Could you check a few things on this model? Use its own coordinates, in mm. Face numbers are marked on the shaded views. A direction names the side the tool comes from. Coordinates: 2 decimals unless noted, no trailing zeros. Loops run counter-clockwise (first coordinate to the right, second up) from the corner with the lowest first, then second, coordinate; pieces in that order, holes last. Notation, with made-up numbers: M 43.25,82.5 L 89.25,82.5 A13 ccw 89.25,86.5 Z; hole C 67,85 d6. An arc over 180 degrees is marked long. Return JSON: item names as keys, results as strings. Group by question number.
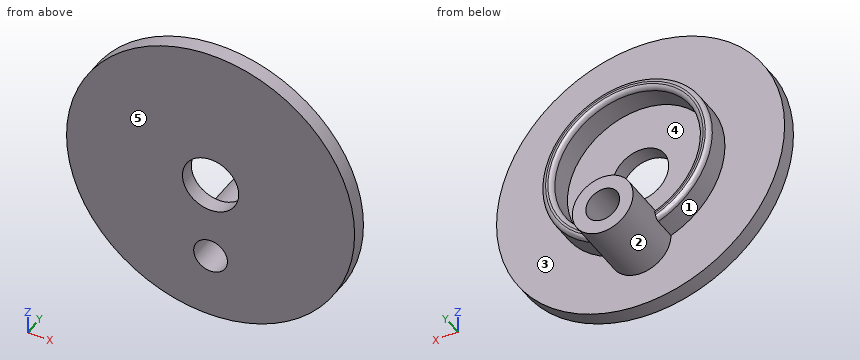
from build123d import *

# Parameters (mm, degrees)
SKETCH2_R           = 64
BOSS_EXTRUDE1_DEPTH = 7
SKETCH3_R           = 37.5
SKETCH3_R_2         = 32.5
BOSS_EXTRUDE2_DEPTH = 12
SKETCH4_R           = 12.5
CUT_EXTRUDE1_DEPTH  = 8
FILLET1_R           = 2
SKETCH5_R           = 13.5
BOSS_EXTRUDE3_DEPTH = 30
SKETCH7_R           = 7.5
CUT_EXTRUDE2_DEPTH  = 38


with BuildPart() as part:
    # Sketch2 → Boss-Extrude1 (new body)
    with BuildSketch(Plane(origin=(0, 0, 0), x_dir=(1, 0, 0), z_dir=(0, 1, 0))):
        Circle(SKETCH2_R)
    extrude(amount=BOSS_EXTRUDE1_DEPTH)

    # Sketch3 → Boss-Extrude2 (add)
    with BuildSketch(Plane(origin=(0, 7, 0), x_dir=(1, 0, 0), z_dir=(0, 1, 0))):
        Circle(SKETCH3_R)
        Circle(SKETCH3_R_2, mode=Mode.SUBTRACT)
    extrude(amount=BOSS_EXTRUDE2_DEPTH)

    # Sketch4 → Cut-Extrude1 (cut, through all)
    with BuildSketch(Plane(origin=(0, 7, 0), x_dir=(1, 0, 0), z_dir=(0, 1, 0))):
        Circle(SKETCH4_R)
    extrude(amount=-CUT_EXTRUDE1_DEPTH, mode=Mode.SUBTRACT)

    # Fillet1
    fillet1_edges = [part.edges().sort_by_distance(p)[0] for p in [
        (-37.5, 19, 0),
        (-32.5, 19, 0),
    ]]
    fillet(fillet1_edges, radius=FILLET1_R)

    # Sketch5 → Boss-Extrude3 (add)
    with BuildSketch(Plane(origin=(0, 7, 0), x_dir=(1, 0, 0), z_dir=(0, 1, 0))):
        with Locations((0, 35)):
            Circle(SKETCH5_R)
    extrude(amount=BOSS_EXTRUDE3_DEPTH)

    # Sketch7 → Cut-Extrude2 (cut, through all)
    with BuildSketch(Plane(origin=(0, 37, 0), x_dir=(1, 0, 0), z_dir=(0, 1, 0))):
        with Locations((0, 35)):
            Circle(SKETCH7_R)
    extrude(amount=-CUT_EXTRUDE2_DEPTH, mode=Mode.SUBTRACT)


solid = part.part
(1) Will these pins go through, and if not, where does the flat tip stop? P1, Ø2, axis at y = 16, z = 28, coming from the +X side; P2, Ø10, axis at y = 16, z = 19, coming from the +X side; P3, Ø1, axis at x = 45, z = 48, coming from the -Y side; P4, Ø10, axis at x = -42, z = 25.5, coming from the +Y side.
(2) Imagine slicing it at C-C, the plane y = 30. Write out the boundary of the cut face in (x, z).
(3) If I drill on L1, parallel to Z at x = 0, y = 16.5; L2, parallel to X at y = 29, z = -35; L3, parallel to X at y = 2.5, z = 0, over which ranges is the centre line in solid material (lowest first)? Write a range as [from, to].
(4) Imagine slicing it at D-D, the plane y = 4.5. Write out the boundary of the cut face in (x, z), then the cut area to 3 significant figures.
(5) For the marked faces 4 and 5, which set-ups out of +Z, -Z, +X, -X, +Y, -Y let a thin tool reach every point of the face, with its end or its side?
(6) We'd pull the mould along Z, two halves only. Please class the marked faces 1, 2 and 3: +Z half, -Z half, draft (parallel to the pull), parting line (faces both ways), or undercut.
(7) Imagine slicing it at A-A, the plane z = 0. Write out the boundary of the cut face in (x, y).
(8) Imagine slicing it at B-B, the plane x = 0. Write out the boundary of the cut face in (y, z).
Checks:
{
 "1": {"P1": "x = 26.02", "P2": "x = 34.79", "P3": "through", "P4": "y = 7"},
 "2": {"outline": "C 0,-35 d27; hole C 0,-35 d15"},
 "3": {"L1": "[-48.5, -42.5], [-27.5, -21.5], [32.5, 37.5]", "L2": "[-13.5, -7.5], [7.5, 13.5]", "L3": "[-64, -12.5], [12.5, 64]"},
 "4": {"outline": "C 0,0 d128; hole C 0,0 d25; hole C 0,-35 d15", "area": "12,200 mm²"},
 "5": {"face 4": "+Y", "face 5": "+Z, -Z, +X, -X, -Y"},
 "6": {"face 1": "parting line", "face 2": "undercut", "face 3": "draft"},
 "7": {"outline": "M -64,0 L -12.5,0 L -12.5,7 L -32.5,7 L -32.5,17 A2 ccw -34.5,19 L -35.5,19 A2 ccw -37.5,17 L -37.5,7 L -64,7 Z; M 12.5,0 L 64,0 L 64,7 L 37.5,7 L 37.5,17 A2 ccw 35.5,19 L 34.5,19 A2 ccw 32.5,17 L 32.5,7 L 12.5,7 Z"},
 "8": {"outline": "M 0,-64 L 7,-64 L 7,-48.5 L 37,-48.5 L 37,-42.5 L 0,-42.5 Z; M 0,-27.5 L 37,-27.5 L 37,-21.5 L 7,-21.5 L 7,-12.5 L 0,-12.5 Z; M 0,12.5 L 7,12.5 L 7,32.5 L 17,32.5 A2 ccw 19,34.5 L 19,35.5 A2 ccw 17,37.5 L 7,37.5 L 7,64 L 0,64 Z"}
}
